```python
from build123d import *

# Parameters (mm, degrees)
SKETCH1_R               = 0.625
BOSS_EXTRUDE1_DEPTH     = 9.5
CUT_EXTRUDE1_DEPTH      = 28.258192056
CUT_EXTRUDE1_DEPTH_BACK = 28.258192056
SKETCH3_R               = 1.325
CUT_EXTRUDE2_START      = -9.5
SKETCH6_R               = 2
CUT_EXTRUDE2_DEPTH      = 2


with BuildPart() as part:
    # Sketch1 → Boss-Extrude1 (new body)
    with BuildSketch(Plane.XY):
        with BuildLine():
            Line((-10.029848506, 2.747640173), (-6.493662943, 7.797836537))
            ThreePointArc((-6.493662943, 7.797836537), (-14.209734002, -10.195642148), (0.059553412, 3.209225046))
            Line((0.059553412, 3.209225046), (-3.476632152, -1.840971318))
            ThreePointArc((-3.476632152, -1.840971318), (-11.34185182, -6.099881927), (-10.029848506, 2.747640173))
        make_face()
        with Locations((-11.114657585, 3.658851871)):
            Circle(SKETCH1_R, mode=Mode.SUBTRACT)
        with Locations((-2.249346687, -2.548705649)):
            Circle(SKETCH1_R, mode=Mode.SUBTRACT)
        with Locations((-12.057904643, -7.122511339)):
            Circle(SKETCH1_R, mode=Mode.SUBTRACT)
    extrude(amount=BOSS_EXTRUDE1_DEPTH)

    # Sketch3 → Cut-Extrude1 (cut, two sides: drawn at the far end of the back side and taken through both)
    with BuildSketch(Plane(origin=(-12.936010228, 9.057891876, 0), x_dir=(0, 0, 1), z_dir=(-0.8191520442889951, 0.5735764363510415, 0)).offset(-CUT_EXTRUDE1_DEPTH_BACK)):
        with Locations(Location((5, -6.519345212, 0), (0, 0, 270))):
            Circle(SKETCH3_R)
    extrude(amount=CUT_EXTRUDE1_DEPTH + CUT_EXTRUDE1_DEPTH_BACK, mode=Mode.SUBTRACT)

    # Sketch6 → Cut-Extrude2 (cut)
    with BuildSketch(Plane(origin=(0, 0, 0), x_dir=(-1, 0, 0), z_dir=(0, 0, -1)).offset(CUT_EXTRUDE2_START)):
        with Locations((11.114657585, 3.658851871)):
            Circle(SKETCH6_R)
        with Locations((12.057904643, -7.122511339)):
            Circle(SKETCH6_R)
        with Locations((2.249346687, -2.548705649)):
            Circle(SKETCH6_R)
    extrude(amount=CUT_EXTRUDE2_DEPTH, mode=Mode.SUBTRACT)


solid = part.part
```
Verification items for the finished model (mm, model axes). A direction names the side the tool comes from. Round coordinates to 2 decimals unless told otherwise and drop trailing zeros. Order: outer loops, then holes, each group sorted by start corner. A loop starts at its lowest first (then second) coordinate and runs counter-clockwise, first axis right, second up. Notation, with made-up numbers: (-34, 67) -> (9, 67) arc R33 cw to (9, 98) -> close; hole circle Ø8 at (1.25, -17). An arc over 180 degrees is marked (long way). Put each result on its own line as item: value. Start each with the question number.
(1) Depth check by flat-ended pin: pin 1 Ø2 at (x, y) = (-12, -7.5) entering from +Z; pin 2 Ø1 at (x, z) = (-4.5, 2.5) entering from +Y; pin 3 Ø5 at (y, z) = (-7, 7) entering from +X. Enter the tip coordinate at first touch or a pass-through.
(2) Section check A-A (z = 5.5). State how many separate pieces and enclosed holes the cut face has, then the cut area to 3 significant figures.
(3) Section check C-C (x = -7.25). Enter the section's corners in (y, z), then the cut area to 3 significant figures.
(4) Draft check along Z on faces 4 (the face through (-8.287, 5.237, 4.684)), 5 (the face through (-1.78, -5.43, 4.19)), 6 (the face through (-12, -8, 7.5)). Enter one of: +Z half, -Z half, draft (parallel to the pull), parting line (faces both ways), or undercut.
(5) Section check B-B (y = -1.5). Enter the section's corners in (x, z), then the cut area to 3 significant figures.
(6) Tool access check on faces 1 (the face through (-14.52, -9.97, 4.68)), 2 (the face through (-1.6, -3, 7.5)), 3 (the face through (-1.684, 0.719, 4.684)). Record the directions out of +Z, -Z, +X, -X, +Y, -Y that give a thin tool (end or side, any length) a straight path to the whole face; none if there is none.
(7) Section check D-D (z = 3.25). Enter the section's corners in (x, y) (3 decimals), then the cut area to 3 significant figures.
(8) Material ranges on line 1 along Y through (x, z) = (-12, 5.25); line 2 along Y through (x, z) = (-2, 4); line 3 along X through (y, z) = (-0.75, 6.25), recorded low to high.
Completed:
1. pin 1: stops at z = 7.5
1. pin 2: stops at y = -4.24
1. pin 3: stops at x = 1.21
2. separate pieces: 3
2. enclosed holes: 3
2. area: 165 mm2
3. outline: (-11.93, 0) -> (-6.85, 0) -> (-6.85, 9.5) -> (-11.93, 9.5) -> close; (6.72, 0) -> (7.92, 0) -> (7.92, 9.5) -> (6.72, 9.5) -> close
3. area: 59.7 mm2
4. face 4: draft
4. face 5: undercut
4. face 6: +Z half
5. outline: (-18.46, 0) -> (-13.45, 0) -> (-13.45, 9.5) -> (-18.46, 9.5) -> close; (-3.24, 0) -> (1.51, 0) -> (1.51, 9.5) -> (-0.55, 9.5) -> (-0.55, 7.5) -> (-3.24, 7.5) -> close
5. area: 87.4 mm2
6. face 1: +Z, -Z
6. face 2: +Z
6. face 3: +Z, -Z, +Y
7. outline: (-10.03, 2.748) -> (-6.494, 7.798) arc R10 ccw (long way) to (0.06, 3.209) -> (-3.477, -1.841) arc R5 cw (long way) to start; hole circle Ø1.25 at (-12.058, -7.123); hole circle Ø1.25 at (-11.115, 3.659); hole circle Ø1.25 at (-2.249, -2.549)
7. area: 189 mm2
8. line 1: y = -11.36 to -7.74, -6.5 to -5.55, 2.03 to 7.35
8. line 2: y = -9.63 to -7.62, -5.5 to -3.12, -1.98 to 0.27
8. line 3: x = -18.4 to -13.31, -2.71 to 1.45
